Source: CAD feature listing. Evaluate the final solid. Frame: model axes, mm. Coordinates: 2 decimals unless noted, no trailing zeros.
```python
from build123d import *

# Parameters (mm, degrees)
SKETCH_1_R      = 1.75
SKETCH_1_R_2    = 2
EXTRUDE_1_DEPTH = 1.5


with BuildPart() as part:
    # Эскиз1 → Бобышка-Вытянуть1 (new body)
    with BuildSketch(Plane(origin=(0, 0, 0), x_dir=(1, 0, 0), z_dir=(0, 1, 0))):
        with BuildLine():
            Line((237.5, 12.5), (237.5, 22))
            Line((237.5, 22), (0, 22))
            Line((0, 22), (0, 0))
            Line((0, 0), (315.5, 0))
            Line((315.5, 0), (315.5, 16))
            Line((315.5, 16), (306.5, 16))
            Line((306.5, 16), (306.5, 12.5))
            ThreePointArc((306.5, 12.5), (305.621320344, 10.378679656), (303.5, 9.5))
            Line((303.5, 9.5), (240.5, 9.5))
            ThreePointArc((240.5, 9.5), (238.378679656, 10.378679656), (237.5, 12.5))
        make_face()
        with Locations((235.5, 7.5)):
            Circle(SKETCH_1_R, mode=Mode.SUBTRACT)
        with Locations((308.5, 7.5)):
            Circle(SKETCH_1_R_2, mode=Mode.SUBTRACT)
        with Locations((15, 16)):
            Circle(SKETCH_1_R, mode=Mode.SUBTRACT)
        with Locations((71, 16)):
            Circle(SKETCH_1_R, mode=Mode.SUBTRACT)
        with Locations((86, 16)):
            Circle(SKETCH_1_R, mode=Mode.SUBTRACT)
        with Locations((142, 16)):
            Circle(SKETCH_1_R, mode=Mode.SUBTRACT)
        with Locations((157, 16)):
            Circle(SKETCH_1_R, mode=Mode.SUBTRACT)
        with Locations((213, 16)):
            Circle(SKETCH_1_R, mode=Mode.SUBTRACT)
    extrude(amount=EXTRUDE_1_DEPTH)


solid = part.part
```
Q1. Material intervals for line 1 along X through (y, z) = (0.7, -7.5); line 2 along X through (y, z) = (0.65, -12.25); line 3 along Z through (x, y) = (213, 1.15), sorted ascending.
Q2. First-contact query: pin 1 Ø3 at (x, z) = (157, -16) entering from +Y; pin 2 Ø0.8 at (x, y) = (310, 1) entering from -Z. Flat tips, straight axial feed; report the tip coordinate or a pass-through.
Q3. Section query A-A on y = 0.25. Count the separate pieces of the cut face and the enclosed holes in it, then the cut area to 3 significant figures.
Resolved:
1. line 1: x = 0 to 233.75, 237.25 to 306.5, 310.5 to 315.5
1. line 2: x = 0 to 237.51, 306.49 to 315.5
1. line 3: z = -22 to -17.75, -14.25 to 0
2. pin 1: passes through
2. pin 2: stops at z = -16
3. separate pieces: 1
3. enclosed holes: 8
3. area: 5,950 mm2
